Model file for the job. Use its own axes, mm. A direction names the side the tool comes from. Round coordinates to 2 decimals unless told otherwise and drop trailing zeros. Write each loop counter-clockwise with the first axis right and the second up, starting at its lowest first coordinate (ties: lowest second). Pieces come first, ordered by that corner, then holes. Notation, with made-up numbers: (17.5, 35) - (50.5, 35) arc R25 cw to (50.5, 47) - close; hole circle Ø7 at (48.5, 15.25). An arc over 180 degrees is marked (long way). One line per item, written item: value.
from build123d import *

# Parameters (mm, degrees)
BOSS_EXTRUDE1_DEPTH = 200


with BuildPart() as part:
    # Sketch1 → Boss-Extrude1 (new body)
    with BuildSketch(Plane(origin=(0, 0, 0), x_dir=(0, 0, -1), z_dir=(1, 0, 0))):
        with BuildLine():
            Line((-20, -25), (-20, -20))
            Line((-20, -20), (-11.547005384, -20))
            Line((-11.547005384, -20), (-4, -6.92820323))
            ThreePointArc((-4, -6.92820323), (0, 8), (4, -6.92820323))
            Line((4, -6.92820323), (11.547005384, -20))
            Line((11.547005384, -20), (20, -20))
            Line((20, -20), (20, -25))
            Line((20, -25), (11.547005384, -25))
            Line((11.547005384, -25), (10.997825762, -24.2))
            Line((10.997825762, -24.2), (-10.997825762, -24.2))
            Line((-10.997825762, -24.2), (-11.547005384, -25))
            Line((-11.547005384, -25), (-20, -25))
        make_face()
    extrude(amount=BOSS_EXTRUDE1_DEPTH)


solid = part.part
1. Band-saw the part on A-A on x = 89. Write the cut outline in (y, z).
Report:
outline: (-25, -20) - (-20, -20) - (-20, -11.55) - (-6.93, -4) arc R8 ccw (long way) to (-6.93, 4) - (-20, 11.55) - (-20, 20) - (-25, 20) - (-25, 11.55) - (-24.2, 11) - (-24.2, -11) - (-25, -11.55) - close
2. Drop flat-ended pins along their axis: pin 1 (9.5 mm diameter, centred on x = 129, z = -16.5, fed in from +Y); pin 2 (9.5 mm diameter, centred on x = 84, z = 16, fed in from +Y); pin 3 (8 mm diameter, centred on x = 113.5, y = 1, fed in from +Z). Give the stop position or say it passes through.
Report:
pin 1: y = -20
pin 2: y = -19.49
pin 3: z = 8
3. Wall check: probe 1 along Y at (x, z) = (59, 0.5); probe 2 along Y at (x, z) = (53, 17.5); probe 3 along Z at (x, y) = (130, -19). Give the ranges that are in metal, low to high. Write a range as [from, to].
Report:
probe 1: [-24.2, 7.98]
probe 2: [-25, -20]
probe 3: [-10.97, 10.97]
4. Band-saw the part on C-C on z = 15. Write the cut outline in (x, y).
Report:
outline: (0, -25) - (200, -25) - (200, -20) - (0, -20) - close
5. Mould opens along Y. For faces 1 (the face through (98.6, -13.37, -7.72)), 2 (the face through (99, -25, 16)), 3 (the face through (99, -20, -16)) say: released by +Y, released by -Y, zero draft, split by the parting line, or undercut.
Report:
face 1: undercut
face 2: released by -Y
face 3: released by +Y
6. Band-saw the part on B-B on y = 0. Write the cut outline in (x, z).
Report:
outline: (0, -8) - (200, -8) - (200, 8) - (0, 8) - close
7. Tool access for faces 4 (the face through (99, -20, 16)), 5 (the face through (98.6, -13.56, 7.83)), 6 (the face through (99, -24.2, 0)): list every direction of +Z, -Z, +X, -X, +Y, -Y with a clear straight run to the whole face (end or side of a thin tool).
Report:
face 4: +Z, +X, -X, +Y
face 5: +Z, +X, -X
face 6: +X, -X, -Y
